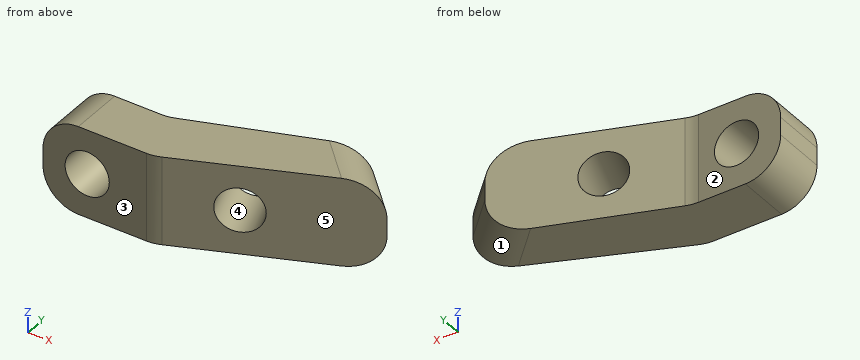
Autodesk Inventor part; units mm, degrees
ref_plane "YZ Plane" through (0, 0, 0) normal (1, 0, 0) x (0, 1, 0)
ref_plane "XZ Plane" through (0, 0, 0) normal (0, 1, 0) x (-1, 0, 0)
ref_plane "XY Plane" through (0, 0, 0) normal (0, 0, 1) x (1, 0, 0)
sketch "Sketch1" plane through (0, 0, 0) normal (0, 0, 1) x (1, 0, 0)
  line L0 (-2.5, -1.5) -> (2.5, -1.5)
  line L1 (2.5, -1.5) -> (2.5, 1.5)
  line L2 (2.5, 1.5) -> (-2.5, 1.5)
  line L3 (-2.5, 1.5) -> (-2.5, -1.5)
  line L4 (-2.5, -1.5) -> (2.5, 1.5) construction
  line L5 (2.5, -1.5) -> (-2.5, 1.5) construction
  line L6 (2.5, 1.5) -> (11.8969, 4.9202)
  line L7 (2.5, 1.5) -> (12.5, 1.5) construction
  line L8 (11.8969, 4.9202) -> (14.0182, 2.7989)
  line L9 (14.0182, 2.7989) -> (3.7426, -1.5)
  line L10 (3.7426, -1.5) -> (2.5, -1.5)
  point P0 (0, 0)
  dimension "d0" = 5
  dimension "d1" = 3
  dimension "d2" = 10
  dimension "d3" = 20
  dimension "d4" = 3
extrude "Extrusion1" add sketch "Sketch1" along normal blind 5
sketch "Sketch2" plane through (-2.5, 1.5, 0) normal (0, 1, 0) x (1, 0, 0)
  line L0 (2.5, 0) -> (2.5, -5)
  line L1 (0, -5) -> (6.2426, -5)
  circle A0 centre (2.5, -2.5) radius 1.25
  dimension "d7" = 2.5
extrude "Extrusion2" cut sketch "Sketch2" against normal blind 5
fillet "Fillet1" radius 2 2 edges at (2.5, 1.5, 2.5) (3.7426, -1.5, 2.5)
sketch "Sketch3" plane through (11.8969, 4.9202, 0) normal (-0.342, 0.9397, 0) x (-0.9397, -0.342, 0)
  line L0 (-1.2679, 0) -> (-1.2679, 5)
  line L1 (-1.2679, 2.5) -> (5.7321, 2.5)
  circle A0 centre (5.7321, 2.5) radius 1.25
  point P0 (12.8623, 0)
  dimension "d11" = 7
  dimension "d12" = 2.5
extrude "Extrusion3" cut sketch "Sketch3" against normal up to next
fillet "Fillet2" radius 2 4 edges at (12.9576, 3.8595, 5) (12.9576, 3.8595, 0) (-2.5, 0, 5) (-2.5, 0, 0)
properties part number "rpi_mount"
Part model, mm, in its own coordinate system. Face numbers are marked on the shaded views. A direction names the side the tool comes from. Round coordinates to 2 decimals unless told otherwise and drop trailing zeros. Loops run counter-clockwise (first coordinate to the right, second up) from the corner with the lowest first, then second, coordinate; pieces in that order, holes last.
Item 1: 3-axis set-ups, long thin cutter, end or side, ignore diameter. For the marked faces 1 and 2: which of +Z, -Z, +X, -X, +Y, -Y reach the whole face in a straight line?
Item 2: Cut at D-D, the plane y = 1. State how many separate pieces and enclosed holes the cut face has, then the cut area to 3 significant figures.
Item 3: Drop flat-ended pins along their axis: P1, Ø1, axis at y = 2, z = 2, coming from the +X side; P2, Ø1.5, axis at y = 1.5, z = 1, coming from the +X side. Give the stop position or say it passes through.
Item 4: Cut at C-C, the plane z = 4.6. Give the cut face in (x, y).
Item 5: Cut at B-B, the plane z = 2.5. Give the cut face in (x, y), then the cut area to 3 significant figures.
Item 6: Drill centre lines: line 1 (Z direction, x = 0, y = -0.6); line 2 (X direction, y = 0.9, z = 2.5); line 3 (Y direction, x = 1.25, z = 2). Where is each one in solid material? Low to high.
Item 7: Mould opens along X. For the marked faces 3, 4 and 5 say: +X half, -X half, draft (parallel to the pull), parting line (faces both ways), or undercut.
Item 8: Cut at A-A, the plane x = 0. Give the cut face in (y, z), then the cut area to 3 significant figures.
A:
1. face 1: -Z, +X, +Y
1. face 2: +Z, -Z, -X, +Y
2. separate pieces: 1
2. enclosed holes: 2
2. area: 49.2 mm2
3. P1: stops at x = 13.3
3. P2: stops at x = 12.71
4. outline: (-1.7, -1.5) - (3.34, -1.5) arc R2 ccw to (4.11, -1.35) - (13.22, 2.47) - (11.07, 4.62) - (2.83, 1.62) arc R2 cw to (2.15, 1.5) - (-1.7, 1.5) - close
5. outline: (-2.5, -1.5) - (-1.25, -1.5) - (-1.25, 1.5) - (-2.5, 1.5) - close; (1.25, -1.5) - (3.34, -1.5) arc R2 ccw to (4.11, -1.35) - (6.4, -0.39) - (5.34, 2.53) - (2.83, 1.62) arc R2 cw to (2.15, 1.5) - (1.25, 1.5) - close; (7.69, 3.39) - (8.71, 0.58) - (14.02, 2.8) - (11.9, 4.92) - close
5. area: 33.4 mm2
6. line 1: z = 0 to 1.25, 3.75 to 5
6. line 2: x = -2.5 to -1.25, 1.25 to 5.93, 8.59 to 9.48
6. line 3: y = -1.5 to 1.5
7. face 3: draft
7. face 4: undercut
7. face 5: +X half
8. outline: (-1.5, 0) - (1.5, 0) - (1.5, 1.25) - (-1.5, 1.25) - close; (-1.5, 3.75) - (1.5, 3.75) - (1.5, 5) - (-1.5, 5) - close
8. area: 7.50 mm2
